Input: part model. Units: mm. Frame: model coordinates. A direction names the side the tool comes from. Give positions to 0.01 mm unless a question says otherwise; leave off trailing zeros. Order: outer loops, then holes, each group sorted by start corner. A loop starts at its lowest first (then second) coordinate and runs counter-clockwise, first axis right, second up. Notation, with made-up numbers: (72, 82) -> (104, 82) arc R22 cw to (104, 94) -> close; hole circle Ø1 at (-1, 58.5). An arc over 180 degrees is marked (long way). Use a Markdown table: item, result. Add a question column.
from build123d import *

# Parameters (mm, degrees)
F1_DEPTH = 3


with BuildPart() as f1:
    # F0 (on Top) → F1 (new body)
    with BuildSketch(Plane.XY):
        Polygon((-81.961524, 107.942286), (-66.961524, 81.961524), (-40.980762, 96.961524), (-55.980762, 122.942286), align=None)
        Polygon((-122.942286, 96.961524), (-107.942286, 122.942286), (-122.942286, 122.942286), align=None)
        Polygon((-122.942286, 66.961524), (-96.961524, 81.961524), (-122.942286, 96.961524), align=None)
        Polygon((-81.961524, 55.980762), (-66.961524, 81.961524), (-81.961524, 107.942286), (-96.961524, 81.961524), align=None)
        Polygon((40.980762, 96.961524), (40.980762, 66.961524), (66.961524, 81.961524), align=None)
        Polygon((-122.942286, -122.942286), (-107.942286, -122.942286), (-122.942286, -96.961524), align=None)
        Polygon((-55.980762, -122.942286), (-81.961524, -107.942286), (-107.942286, -122.942286), align=None)
        Polygon((-81.961524, -107.942286), (-66.961524, -81.961524), (-81.961524, -55.980762), (-96.961524, -81.961524), align=None)
        Polygon((-96.961524, -81.961524), (-81.961524, -55.980762), (-107.942286, -40.980762), (-122.942286, -66.961524), align=None)
        Polygon((-40.980762, -96.961524), (-40.980762, -66.961524), (-66.961524, -81.961524), align=None)
        Polygon((-66.961524, -81.961524), (-40.980762, -66.961524), (-55.980762, -40.980762), (-81.961524, -55.980762), align=None)
        Polygon((-40.980762, -15), (-15, 0), (-40.980762, 15), align=None)
        Polygon((-96.961524, 0), (-81.961524, 25.980762), (-107.942286, 40.980762), (-122.942286, 15), align=None)
        Polygon((-81.961524, -25.980762), (-66.961524, 0), (-81.961524, 25.980762), (-96.961524, 0), align=None)
        Polygon((-122.942286, -15), (-96.961524, 0), (-122.942286, 15), align=None)
        Polygon((-107.942286, 40.980762), (-81.961524, 55.980762), (-96.961524, 81.961524), (-122.942286, 66.961524), align=None)
        Polygon((-122.942286, 15), (-107.942286, 40.980762), (-122.942286, 66.961524), align=None)
        Polygon((-96.961524, 81.961524), (-81.961524, 107.942286), (-107.942286, 122.942286), (-122.942286, 96.961524), align=None)
        Polygon((-81.961524, 25.980762), (-55.980762, 40.980762), (-81.961524, 55.980762), align=None)
        Polygon((40.980762, 66.961524), (55.980762, 40.980762), (81.961524, 55.980762), (66.961524, 81.961524), align=None)
        Polygon((0, 55.980762), (25.980762, 40.980762), (40.980762, 66.961524), (15, 81.961524), align=None)
        Polygon((66.961524, 81.961524), (81.961524, 55.980762), (96.961524, 81.961524), (81.961524, 107.942286), align=None)
        Polygon((15, 81.961524), (40.980762, 66.961524), (40.980762, 96.961524), align=None)
        Polygon((-15, -81.961524), (-40.980762, -66.961524), (-40.980762, -96.961524), align=None)
        Polygon((-40.980762, -96.961524), (-66.961524, -81.961524), (-81.961524, -107.942286), (-55.980762, -122.942286), align=None)
        Polygon((0, -55.980762), (-25.980762, -40.980762), (-40.980762, -66.961524), (-15, -81.961524), align=None)
        Polygon((-40.980762, -66.961524), (-25.980762, -40.980762), (-40.980762, -15), (-55.980762, -40.980762), align=None)
        Polygon((-81.961524, -55.980762), (-55.980762, -40.980762), (-81.961524, -25.980762), align=None)
        Polygon((-107.942286, -122.942286), (-81.961524, -107.942286), (-96.961524, -81.961524), (-122.942286, -96.961524), align=None)
        Polygon((-122.942286, -96.961524), (-96.961524, -81.961524), (-122.942286, -66.961524), align=None)
        Polygon((25.980762, -122.942286), (0, -107.942286), (-25.980762, -122.942286), align=None)
        Polygon((40.980762, -96.961524), (15, -81.961524), (0, -107.942286), (25.980762, -122.942286), align=None)
        Polygon((0, -107.942286), (-15, -81.961524), (-40.980762, -96.961524), (-25.980762, -122.942286), align=None)
        Polygon((-25.980762, -122.942286), (-40.980762, -96.961524), (-55.980762, -122.942286), align=None)
        Polygon((-55.980762, 122.942286), (-40.980762, 96.961524), (-25.980762, 122.942286), align=None)
        Polygon((-25.980762, 122.942286), (0, 107.942286), (25.980762, 122.942286), align=None)
        Polygon((0, 107.942286), (15, 81.961524), (40.980762, 96.961524), (25.980762, 122.942286), align=None)
        Polygon((-40.980762, 96.961524), (-15, 81.961524), (0, 107.942286), (-25.980762, 122.942286), align=None)
        Polygon((40.980762, 96.961524), (66.961524, 81.961524), (81.961524, 107.942286), (55.980762, 122.942286), align=None)
        Polygon((25.980762, 122.942286), (40.980762, 96.961524), (55.980762, 122.942286), align=None)
        Polygon((55.980762, 122.942286), (81.961524, 107.942286), (107.942286, 122.942286), align=None)
        Polygon((107.942286, 122.942286), (122.942286, 96.961524), (122.942286, 122.942286), align=None)
        Polygon((0, -55.980762), (0, -25.980762), (-25.980762, -40.980762), align=None)
        Polygon((81.961524, 107.942286), (96.961524, 81.961524), (122.942286, 96.961524), (107.942286, 122.942286), align=None)
        Polygon((-107.942286, 40.980762), (-81.961524, 25.980762), (-81.961524, 55.980762), align=None)
        Polygon((-122.942286, -66.961524), (-107.942286, -40.980762), (-122.942286, -15), align=None)
        Polygon((-66.961524, 81.961524), (-40.980762, 66.961524), (-40.980762, 96.961524), align=None)
        Polygon((-81.961524, -55.980762), (-81.961524, -25.980762), (-107.942286, -40.980762), align=None)
        Polygon((-107.942286, -40.980762), (-81.961524, -25.980762), (-96.961524, 0), (-122.942286, -15), align=None)
        Polygon((122.942286, -66.961524), (96.961524, -81.961524), (122.942286, -96.961524), align=None)
        Polygon((122.942286, -96.961524), (96.961524, -81.961524), (81.961524, -107.942286), (107.942286, -122.942286), align=None)
        Polygon((66.961524, -81.961524), (40.980762, -66.961524), (40.980762, -96.961524), align=None)
        Polygon((81.961524, -55.980762), (55.980762, -40.980762), (40.980762, -66.961524), (66.961524, -81.961524), align=None)
        Polygon((-40.980762, 96.961524), (-40.980762, 66.961524), (-15, 81.961524), align=None)
        Polygon((40.980762, -96.961524), (40.980762, -66.961524), (15, -81.961524), align=None)
        Polygon((107.942286, -122.942286), (81.961524, -107.942286), (55.980762, -122.942286), align=None)
        Polygon((-15, 81.961524), (0, 55.980762), (15, 81.961524), (0, 107.942286), align=None)
        Polygon((55.980762, -122.942286), (40.980762, -96.961524), (25.980762, -122.942286), align=None)
        Polygon((0, -25.980762), (15, 0), (0, 25.980762), (-15, 0), align=None)
        Polygon((0, 25.980762), (15, 0), (40.980762, 15), (25.980762, 40.980762), align=None)
        Polygon((122.942286, 96.961524), (96.961524, 81.961524), (122.942286, 66.961524), align=None)
        Polygon((25.980762, 40.980762), (40.980762, 15), (55.980762, 40.980762), (40.980762, 66.961524), align=None)
        Polygon((25.980762, -40.980762), (0, -25.980762), (0, -55.980762), align=None)
        Polygon((96.961524, 0), (81.961524, -25.980762), (107.942286, -40.980762), (122.942286, -15), align=None)
        Polygon((66.961524, 0), (40.980762, 15), (40.980762, -15), align=None)
        Polygon((122.942286, 66.961524), (107.942286, 40.980762), (122.942286, 15), align=None)
        Polygon((55.980762, -40.980762), (40.980762, -15), (25.980762, -40.980762), (40.980762, -66.961524), align=None)
        Polygon((81.961524, 25.980762), (66.961524, 0), (81.961524, -25.980762), (96.961524, 0), align=None)
        Polygon((40.980762, -15), (15, 0), (0, -25.980762), (25.980762, -40.980762), align=None)
        Polygon((122.942286, -122.942286), (122.942286, -96.961524), (107.942286, -122.942286), align=None)
        Polygon((-15, 0), (0, 25.980762), (-25.980762, 40.980762), (-40.980762, 15), align=None)
        Polygon((-25.980762, 40.980762), (0, 25.980762), (0, 55.980762), align=None)
        Polygon((107.942286, 40.980762), (81.961524, 25.980762), (96.961524, 0), (122.942286, 15), align=None)
        Polygon((122.942286, 15), (96.961524, 0), (122.942286, -15), align=None)
        Polygon((66.961524, 0), (40.980762, -15), (55.980762, -40.980762), (81.961524, -25.980762), align=None)
        Polygon((55.980762, 40.980762), (40.980762, 15), (66.961524, 0), (81.961524, 25.980762), align=None)
        Polygon((15, -81.961524), (0, -55.980762), (-15, -81.961524), (0, -107.942286), align=None)
        Polygon((0, 55.980762), (0, 25.980762), (25.980762, 40.980762), align=None)
        Polygon((96.961524, 81.961524), (81.961524, 55.980762), (107.942286, 40.980762), (122.942286, 66.961524), align=None)
        Polygon((81.961524, 55.980762), (55.980762, 40.980762), (81.961524, 25.980762), align=None)
        Polygon((81.961524, -25.980762), (55.980762, -40.980762), (81.961524, -55.980762), (107.942286, -40.980762), align=None)
        Polygon((81.961524, 55.980762), (81.961524, 25.980762), (107.942286, 40.980762), align=None)
        Polygon((122.942286, -15), (107.942286, -40.980762), (122.942286, -66.961524), align=None)
        Polygon((-40.980762, 66.961524), (-25.980762, 40.980762), (0, 55.980762), (-15, 81.961524), align=None)
        Polygon((107.942286, -40.980762), (81.961524, -55.980762), (96.961524, -81.961524), (122.942286, -66.961524), align=None)
        Polygon((96.961524, -81.961524), (81.961524, -55.980762), (66.961524, -81.961524), (81.961524, -107.942286), align=None)
        Polygon((81.961524, -107.942286), (66.961524, -81.961524), (40.980762, -96.961524), (55.980762, -122.942286), align=None)
        Polygon((-25.980762, -40.980762), (0, -25.980762), (-15, 0), (-40.980762, -15), align=None)
        Polygon((-55.980762, 40.980762), (-40.980762, 66.961524), (-66.961524, 81.961524), (-81.961524, 55.980762), align=None)
        Polygon((-40.980762, 15), (-25.980762, 40.980762), (-40.980762, 66.961524), (-55.980762, 40.980762), align=None)
        Polygon((40.980762, 15), (15, 0), (40.980762, -15), align=None)
        Polygon((40.980762, -66.961524), (25.980762, -40.980762), (0, -55.980762), (15, -81.961524), align=None)
        Polygon((-40.980762, -15), (-40.980762, 15), (-66.961524, 0), align=None)
        Polygon((-55.980762, -40.980762), (-40.980762, -15), (-66.961524, 0), (-81.961524, -25.980762), align=None)
        Polygon((-66.961524, 0), (-40.980762, 15), (-55.980762, 40.980762), (-81.961524, 25.980762), align=None)
    extrude(amount=F1_DEPTH)


solid = f1.part
Q1. Ray query, line 1 (Y direction, x = -65, z = 2.25); line 2 (Y direction, x = -72, z = 1.8). Return the intervals inside material, ascending.
Q2. Access query for faces 1 (the flat face through (-2, 2, 3)), 2 (the flat face through (-94.77, 115.337, 1.479)). Directions: +Z, -Z, +X, -X, +Y, -Y. A direction counts if a zero-diameter tool reaches every point of the face in a straight line with its end or side. Return the directions, or none.
Q3. Draft query along X for faces 3 (the flat face through (-2, 2, 0)), 4 (the flat face through (-68.789, 115.547, 1.479)). Return one class per face: +X half, -X half, draft (parallel to the pull), parting line (faces both ways), or undercut.
Q4. Section query A-A (x = -90.5). Return loops of the section in (y, z).
Solution:
| question | item | result |
|---|---|---|
| 1 | line 1 | y = -122.94 to 117.74 |
| 1 | line 2 | y = -122.94 to 113.69 |
| 2 | face 1 | +Z, +X, -X, +Y, -Y |
| 2 | face 2 | +Z, -Z, +Y |
| 3 | face 3 | draft |
| 3 | face 4 | undercut |
| 4 | outline | (-122.94, 0) -> (112.87, 0) -> (112.87, 3) -> (-122.94, 3) -> close |
